Autodesk Inventor part; units mm, degrees
ref_plane "YZ Plane" through (0, 0, 0) normal (1, 0, 0) x (0, 1, 0)
ref_plane "XZ Plane" through (0, 0, 0) normal (0, 1, 0) x (-1, 0, 0)
ref_plane "XY Plane" through (0, 0, 0) normal (0, 0, 1) x (1, 0, 0)
sketch "Sketch1" plane through (0, 0, 0) normal (0, 0, 1) x (1, 0, 0)
  circle A0 centre (0, 0) radius 93
  circle A1 centre (0, 0) radius 85
  dimension "d0" = 186
  dimension "d1" = 170
extrude "Extrusion1" add sketch "Sketch1" along normal blind 38
fillet "Fillet1" radius 2 3 edges at (-85, 0, 38) (-85, 0, 0) (-93, 0, 0)
properties part number "Flywheel outer rim" material "Steel, Carbon"
Can you work these out from the model? Positions are in its coordinate system, mm. Give positions to 0.01 mm unless a question says otherwise; leave off trailing zeros. Loops run counter-clockwise (first coordinate to the right, second up) from the corner with the lowest first, then second, coordinate; pieces in that order, holes last. Notation, with made-up numbers: (57.5, 54.5) - (111.5, 54.5) arc R37 ccw to (111.5, 92.5) - close; hole circle Ø2 at (64, 39.25). An arc over 180 degrees is marked (long way). Answer as a JSON object with one key per item and string values.
Q1. If I drill on L1, parallel to Y at x = 0, z = 19; L2, parallel to X at y = -61, z = 3; L3, parallel to X at y = 72, z = 10.5, over which ranges is the centre line in solid material (lowest first)?
Geometry says:
{"L1": "-93 to -85, 85 to 93", "L2": "-70.2 to -59.19, 59.19 to 70.2", "L3": "-58.86 to -45.18, 45.18 to 58.86"}
Q2. If we mould it in two halves opening along X, with no side actions, what happens to faces 1 (the cylindrical face through (88.705, -27.935, 19.748)), 2 (the flat face through (47, -74, 0)), 3 (the cylindrical face through (-67.453, 51.721, 18.762))? For each: pulls with the +X half, pulls with the -X half, needs draft (parallel to the pull), parting line crosses it, or undercut.
Geometry says:
{"face 1": "parting line crosses it", "face 2": "needs draft", "face 3": "undercut"}
Q3. Will these pins go through, and if not, where does the flat tip stop? P1, Ø4, axis at y = -58, z = 24.5, coming from the -X side; P2, Ø8, axis at y = -35.5, z = 13, coming from the +X side; P3, Ø1, axis at y = 1, z = 12, coming from the +X side.
Geometry says:
{"P1": "x = -74.25", "P2": "x = 87.5", "P3": "x = 93"}
Q4. Imagine slicing it at C-C on z = 14. Write out the boundary of the cut face in (x, y).
Geometry says:
{"outline": "circle Ø186 at (0, 0); hole circle Ø170 at (0, 0)"}
Q5. Imagine slicing it at A-A on y = 0. Write out the boundary of the cut face in (x, z), plus the area to 3 significant figures.
Geometry says:
{"outline": "(-93, 2) arc R2 ccw to (-91, 0) - (-87, 0) arc R2 ccw to (-85, 2) - (-85, 36) arc R2 ccw to (-87, 38) - (-93, 38) - close; (85, 2) arc R2 ccw to (87, 0) - (91, 0) arc R2 ccw to (93, 2) - (93, 38) - (87, 38) arc R2 ccw to (85, 36) - close", "area": "603 mm²"}
